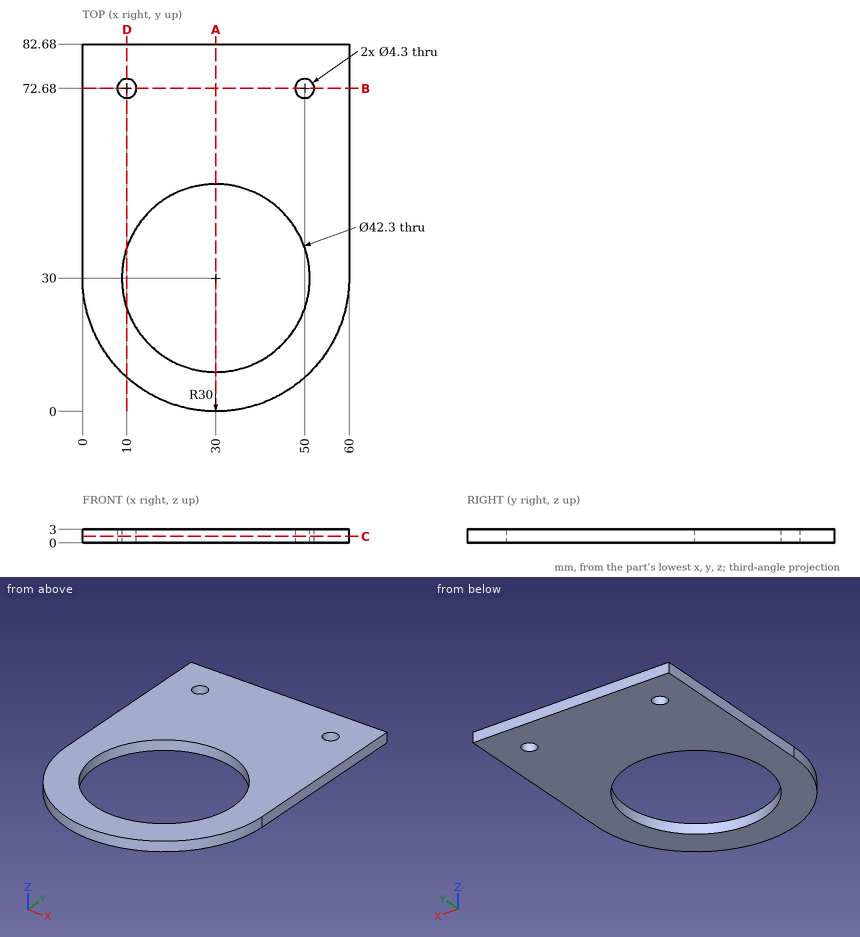
Geometry check sheet. Reference: drawing and pictorial views, mm from the part's lowest x, y, z. Give positions to 0.01 mm unless a question says otherwise; leave off trailing zeros. Order: outer loops, then holes, each group sorted by start corner. A loop starts at its lowest first (then second) coordinate and runs counter-clockwise, first axis right, second up.
1. Section check B-B, the plane y = 72.68. Enter the section's corners in (x, z).
2. Section check A-A, the plane x = 30. Enter the section's corners in (y, z), and give its area (3 significant figures).
3. Section check D-D, the plane x = 10. Enter the section's corners in (y, z), and give its area (3 significant figures).
4. Section check C-C, the plane z = 1.4. Enter the section's corners in (x, y).
5. Gauge pin test, flat end, axial feed: pin 1 Ø7 at (x, y) = (10, 72.68) entering from +Z. Record the tip position at first contact, or that the pin passes through.
6. Thickness scan on L1, parallel to X at y = 72.68, z = 1.2; L2, parallel to Y at x = 29.5, z = 1.2; L3, parallel to X at y = 74.5, z = 1.25. Record the ranges inside material, lowest first.
Values follow:
1. outline: (0, 0) - (7.85, 0) - (7.85, 3) - (0, 3) - close; (12.15, 0) - (47.85, 0) - (47.85, 3) - (12.15, 3) - close; (52.15, 0) - (60, 0) - (60, 3) - (52.15, 3) - close
2. outline: (0, 0) - (8.85, 0) - (8.85, 3) - (0, 3) - close; (51.15, 0) - (82.68, 0) - (82.68, 3) - (51.15, 3) - close
2. area: 121 mm2
3. outline: (7.64, 0) - (23.12, 0) - (23.12, 3) - (7.64, 3) - close; (36.88, 0) - (70.53, 0) - (70.53, 3) - (36.88, 3) - close; (74.83, 0) - (82.68, 0) - (82.68, 3) - (74.83, 3) - close
3. area: 171 mm2
4. outline: (0, 30) arc R30 ccw to (60, 30) - (60, 82.68) - (0, 82.68) - close; hole circle Ø4.3 at (10, 72.68); hole circle Ø42.3 at (30, 30); hole circle Ø4.3 at (50, 72.68)
5. pin 1: stops at z = 3
6. L1: x = 0 to 7.85, 12.15 to 47.85, 52.15 to 60
6. L2: y = 0 to 8.86, 51.14 to 82.68
6. L3: x = 0 to 8.86, 11.14 to 48.86, 51.14 to 60
